For this review, take the finished solid that the model builds, in its own axes (mm). A direction names the side the tool comes from. Round coordinates to 2 decimals unless told otherwise and drop trailing zeros. Write each loop counter-clockwise with the first axis right and the second up, starting at its lowest first coordinate (ties: lowest second). Pieces come first, ordered by that corner, then holes. Notation, with made-up numbers: (-38, 11) -> (-26, 11) arc R8 cw to (-26, 19) -> close; hole circle Ø5 at (-9.75, 51). An arc over 180 degrees is marked (long way). Answer in a Markdown table with one row per item. Add a question column.
```python
from build123d import *

# Parameters (mm, degrees)
EXTRUDE_1_DEPTH        = 20
EXTRUDE_2_DEPTH        = 70
F_1_4_BASE_D           = 3.4
F_1_4_BASE_CBORE_D     = 6.7
F_1_4_BASE_CBORE_DEPTH = 1.65
SKETCH_11_W            = 22
SKETCH_11_H            = 42
CUT_EXTRUDE_1_DEPTH    = 32
CUT_EXTRUDE_2_DEPTH    = 67
CUT_EXTRUDE_3_DEPTH    = 2
CUT_EXTRUDE_4_DEPTH    = 3.5


with BuildPart() as part:
    # 草图1 → 凸台-拉伸1 (new body)
    with BuildSketch(Plane(origin=(0, 0, 0), x_dir=(1, 0, 0), z_dir=(0, 1, 0))):
        with BuildLine():
            Line((75.055476805, 35), (35.707142143, 35))
            ThreePointArc((35.707142143, 35), (46.289075964, 18.902948088), (50, 0))
            ThreePointArc((50, 0), (46.289075964, -18.902948088), (35.707142143, -35))
            Line((35.707142143, -35), (75.055476805, -35))
            Line((75.055476805, -35), (75.055476805, 35))
        make_face()
        with BuildLine():
            Line((0.055476805, -35), (0.055476805, 35))
            Line((0.055476805, 35), (35.707142143, 35))
            ThreePointArc((35.707142143, 35), (-50, 0), (35.707142143, -35))
            Line((35.707142143, -35), (0.055476805, -35))
        make_face()
        with BuildLine():
            Line((35.707142143, 35), (0.055476805, 35))
            Line((0.055476805, 35), (0.055476805, -35))
            Line((0.055476805, -35), (35.707142143, -35))
            ThreePointArc((35.707142143, -35), (46.289075964, -18.902948088), (50, 0))
            ThreePointArc((50, 0), (46.289075964, 18.902948088), (35.707142143, 35))
        make_face()
    extrude(amount=EXTRUDE_1_DEPTH)

    # 草图2 → 凸台-拉伸2 (add)
    with BuildSketch(Plane.XY.offset(35)):
        Polygon((75.055476805, 0), (140.174133177, 114.192122372), (140.174133177, 191.411564081), (120.174133177, 191.411564081), (120.174133177, 109.286292207), (75.055476805, 20), align=None)
    extrude(amount=-EXTRUDE_2_DEPTH)

    # 1/4 六角头螺钉的柱形沉头孔base (through all)
    with Locations(Plane(origin=(0, 20, 0), x_dir=(1, 0, 0), z_dir=(0, 1, 0))):
        with Locations((0, 0)):
            CounterBoreHole(F_1_4_BASE_D / 2, F_1_4_BASE_CBORE_D / 2, F_1_4_BASE_CBORE_DEPTH)

    # 草图11 → 切除-拉伸1 (cut)
    with BuildSketch(Plane(origin=(140.174133177, 0, 0), x_dir=(0, 0, -1), z_dir=(1, 0, 0))):
        with Locations((0, 152.801564081)):
            Rectangle(SKETCH_11_W, SKETCH_11_H)
    extrude(amount=-CUT_EXTRUDE_1_DEPTH, mode=Mode.SUBTRACT)

    # 草图14 → 切除-拉伸2 (cut)
    with BuildSketch(Plane(origin=(140.174133177, 0, 0), x_dir=(0, 0, -1), z_dir=(1, 0, 0))):
        with BuildLine():
            Line((-10, 179.101564081), (10, 179.101564081))
            ThreePointArc((10, 179.101564081), (11, 178.101564081), (10, 177.101564081))
            Line((10, 177.101564081), (-10, 177.101564081))
            ThreePointArc((-10, 177.101564081), (-11, 178.101564081), (-10, 179.101564081))
        make_face()
        with BuildLine():
            Line((-10, 128.501564081), (8.706275956, 128.501564081))
            ThreePointArc((8.706275956, 128.501564081), (9.706275956, 127.501564081), (8.706275956, 126.501564081))
            Line((8.706275956, 126.501564081), (-10, 126.501564081))
            ThreePointArc((-10, 126.501564081), (-11, 127.501564081), (-10, 128.501564081))
        make_face()
    extrude(amount=-CUT_EXTRUDE_2_DEPTH, mode=Mode.SUBTRACT)

    # 草图19 → 切除-拉伸3 (cut)
    with BuildSketch(Plane.XZ):
        with BuildLine():
            Line((-29.938978194, 2.983548036), (0, 6))
            Line((0, 6), (29.925496738, 2.977040035))
            ThreePointArc((29.925496738, 2.977040035), (32.999946297, -0.039985046), (29.889613095, -3.020003134))
            Line((29.889613095, -3.020003134), (0, -6))
            Line((0, -6), (-30.07371717, -4.263466486))
            ThreePointArc((-30.07371717, -4.263466486), (-33.623512821, -0.572707651), (-29.938978194, 2.983548036))
        make_face()
    extrude(amount=-CUT_EXTRUDE_3_DEPTH, mode=Mode.SUBTRACT)

    # 草图20 → 切除-拉伸4 (cut)
    with BuildSketch(Plane.XZ):
        Polygon((0, 6), (-10.447108364, 4.947418969), (-10.447108364, -5.396757185), (0, -6), (10.446834114, -4.958449786), (10.446834114, 4.944700515), align=None)
    extrude(amount=-CUT_EXTRUDE_4_DEPTH, mode=Mode.SUBTRACT)


solid = part.part
```
1. The part is to be moulded in two halves that separate along X. For faces 1 (the cylindrical face through (-3.347, 19.187, -0.147)), 2 (the flat face through (107, 82, -35)), 3 (the cylindrical face through (-49.973, 9.86, -1.656)), say which applies: pulls with the +X half, pulls with the -X half, needs draft (parallel to the pull), parting line crosses it, or undercut.
2. We need section A-A (x = 127.5). Write out the cut boundary in (y, z).
3. We need section B-B (z = 20.5). Write out the cut boundary in (x, y), plus the area to 3 significant figures.
4. We need section D-D (y = 55.5). Write out the cut boundary in (x, z).
5. Tool access review of faces 4 (the flat face through (-22, 2, 0)), 5 (the flat face through (130, 153, 11)), 6 (the flat face through (120.174, 151, 16)), 7 (the flat face through (107, 82, 35)): name each direction out of +Z, -Z, +X, -X, +Y, -Y from which nothing blocks a thin tool from reaching the whole face with its end or side.
6. Clearance check with flat-ended pins moving along their axes: pin 1 Ø16 at (x, z) = (131, 3) entering from -Y; pin 2 Ø22 at (x, z) = (126, -2) entering from -Y; pin 3 Ø1 at (x, z) = (-3, 24.5) entering from +Y. State where each tip first meets the part, or that it passes through.
7. We need section C-C (x = 27). Write out the cut boundary in (y, z).
8. For L1, parallel to Z at x = 0, y = 10.5; L2, parallel to Z at x = 0, y = 19; L3, parallel to Y at x = 73.5, z = 16, list the stretches that pass through material, from the lowest coordinate up. Write a range as [from, to].
Response:
| question | item | result |
|---|---|---|
| 1 | face 1 | undercut |
| 1 | face 2 | needs draft |
| 1 | face 3 | parting line crosses it |
| 2 | outline | (91.97, -35) -> (191.41, -35) -> (191.41, 35) -> (91.97, 35) -> close; hole (126.5, -8.71) arc R1 ccw to (128.5, -8.71) -> (128.5, 10) arc R1 ccw to (126.5, 10) -> close; hole (131.8, -11) -> (173.8, -11) -> (173.8, 11) -> (131.8, 11) -> close; hole (177.1, -10) arc R1 ccw to (179.1, -10) -> (179.1, 10) arc R1 ccw to (177.1, 10) -> close |
| 3 | outline | (-45.6, 0) -> (75.06, 0) -> (140.17, 114.19) -> (140.17, 191.41) -> (120.17, 191.41) -> (120.17, 109.29) -> (75.06, 20) -> (-45.6, 20) -> close |
| 3 | area | 5,440 mm2 |
| 4 | outline | (92.99, -35) -> (106.7, -35) -> (106.7, 35) -> (92.99, 35) -> close |
| 5 | face 4 | -Y |
| 5 | face 5 | +X, -X |
| 5 | face 6 | +Z, -Z, -X, +Y |
| 5 | face 7 | +Z, +X, +Y, -Y |
| 6 | pin 1 | y = 84.08 |
| 6 | pin 2 | y = 70.05 |
| 6 | pin 3 | y = 20 |
| 7 | outline | (0, -42.08) -> (20, -42.08) -> (20, 42.08) -> (0, 42.08) -> (0, 3.27) -> (2, 3.27) -> (2, -3.31) -> (0, -3.31) -> close |
| 8 | L1 | [-50, -1.7], [1.7, 50] |
| 8 | L2 | [-50, -3.35], [3.35, 50] |
| 8 | L3 | [0, 20] |
